```python
from build123d import *

# Parameters (mm, degrees)
SKETCH1_R                               = 87.47125
BOSS_EXTRUDE1_DEPTH                     = 25.4
BOSS_EXTRUDE2_DEPTH                     = 25.4
CUT_EXTRUDE1_REACH                      = 31.21
CUT_EXTRUDE1_START                      = -3.81
SKETCH8_R                               = 72.38365
CBORE_FOR_M6_HEX_HEAD_BOLT1_D           = 7
CBORE_FOR_M6_HEX_HEAD_BOLT1_CBORE_D     = 14.547
CBORE_FOR_M6_HEX_HEAD_BOLT1_CBORE_DEPTH = 4


with BuildPart() as part:
    # Sketch1 → Boss-Extrude1 (new body)
    with BuildSketch(Plane.XY):
        Circle(SKETCH1_R)
    extrude(amount=BOSS_EXTRUDE1_DEPTH)

    # Sketch3 → Boss-Extrude2 (add)
    with BuildSketch(Plane.XY):
        with BuildLine():
            ThreePointArc((-76.246005737, 105.719498865), (-102.262666579, 102.262666579), (-105.719498865, 76.246005737))
            ThreePointArc((-105.719498865, 76.246005737), (-92.490752346, 39.105377809), (-87.47125, 0))
            ThreePointArc((-87.47125, 0), (-92.490752346, -39.105377809), (-105.719498865, -76.246005737))
            ThreePointArc((-105.719498865, -76.246005737), (-102.262666579, -102.262666579), (-76.246005737, -105.719498865))
            ThreePointArc((-76.246005737, -105.719498865), (-39.105377809, -92.490752346), (0, -87.47125))
            ThreePointArc((0, -87.47125), (39.105377809, -92.490752346), (76.246005737, -105.719498865))
            ThreePointArc((76.246005737, -105.719498865), (102.262666579, -102.262666579), (105.719498865, -76.246005737))
            ThreePointArc((105.719498865, -76.246005737), (92.490752346, -39.105377809), (87.47125, 0))
            ThreePointArc((87.47125, 0), (92.490752346, 39.105377809), (105.719498865, 76.246005737))
            ThreePointArc((105.719498865, 76.246005737), (102.262666579, 102.262666579), (76.246005737, 105.719498865))
            ThreePointArc((76.246005737, 105.719498865), (39.105377809, 92.490752346), (0, 87.47125))
            ThreePointArc((0, 87.47125), (-39.105377809, 92.490752346), (-76.246005737, 105.719498865))
        make_face()
    extrude(amount=BOSS_EXTRUDE2_DEPTH)

    # Sketch8 → Cut-Extrude1 (cut, up to next)
    with BuildSketch(Plane.XY.offset(25.4).offset(CUT_EXTRUDE1_START), mode=Mode.PRIVATE) as cut_extrude1_sk1:
        Circle(SKETCH8_R)
    cut_extrude1_tool1 = extrude(cut_extrude1_sk1.sketch, amount=-CUT_EXTRUDE1_REACH, mode=Mode.PRIVATE) & part.part
    add(cut_extrude1_tool1.solids().sort_by_distance((0, 0, 21.59))[0], mode=Mode.SUBTRACT)

    # CBORE for M6 Hex Head Bolt1 (through all)
    with Locations(Plane.XY.offset(25.4)):
        with Locations((-86.996231173, 86.996231173), (86.996231173, 86.996231173), (86.996231173, -86.996231173), (-86.996231173, -86.996231173)):
            CounterBoreHole(CBORE_FOR_M6_HEX_HEAD_BOLT1_D / 2, CBORE_FOR_M6_HEX_HEAD_BOLT1_CBORE_D / 2, CBORE_FOR_M6_HEX_HEAD_BOLT1_CBORE_DEPTH)


solid = part.part
```
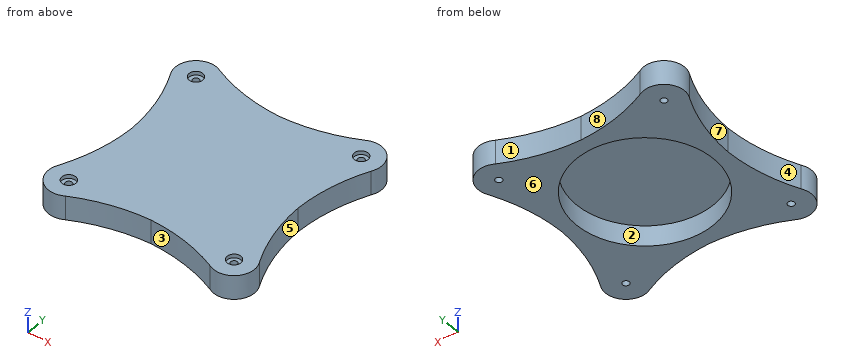
Design review of the part built by this model. Coordinates are the model's own, in mm. Face numbers are marked on the shaded views. A direction names the side the tool comes from. Coordinates: 2 decimals unless noted, no trailing zeros. Loops run counter-clockwise (first coordinate to the right, second up) from the corner with the lowest first, then second, coordinate; pieces in that order, holes last.
Q1. We need section B-B on x = 14.5. State the section outline as (y, z) points, and give its area (3 significant figures).
Reported:
outline: (-88.34, 0) - (-70.92, 0) - (-70.92, 21.59) - (70.92, 21.59) - (70.92, 0) - (88.34, 0) - (88.34, 25.4) - (-88.34, 25.4) - close
area: 1,430 mm2
Q2. We need section A-A on y = 5. State the section outline as (x, z) points, and give its area (3 significant figures).
Reported:
outline: (-87.64, 0) - (-72.21, 0) - (-72.21, 21.59) - (72.21, 21.59) - (72.21, 0) - (87.64, 0) - (87.64, 25.4) - (-87.64, 25.4) - close
area: 1,330 mm2
Q3. Tool access review of the marked faces 1, 2, 3, 4 and 5: name each direction out of +Z, -Z, +X, -X, +Y, -Y from which nothing blocks a thin tool from reaching the whole face with its end or side.
Reported:
face 1: +Z, -Z, +Y
face 2: -Z
face 3: +Z, -Z, -Y
face 4: +Z, -Z, -X
face 5: +Z, -Z, +X
Q4. To check wall thickness, follow line 1 (Z direction, x = -3, y = 1.5); line 2 (Y direction, x = 26.5, z = 14.5); line 3 (X direction, y = 58.5, z = 6). State the ranges of each line that lie inside material, in increasing order.
Reported:
line 1: z = 21.59 to 25.4
line 2: y = -89.94 to -67.36, 67.36 to 89.94
line 3: x = -98.28 to -42.63, 42.63 to 98.28
Q5. For pin 1 (1.5 mm diameter, centred on y = -11, z = 9.5, fed in from -X); pin 2 (5 mm diameter, centred on x = -26.5, z = 3, fed in from +Y); pin 3 (8 mm diameter, centred on x = 87, y = -87, fed in from +Z), all flat-tipped, find the tip position at first contact; note any pin that passes through.
Reported:
pin 1: stops at x = -88.09
pin 2: stops at y = 90.37
pin 3: stops at z = 21.4
Q6. The part is to be moulded in two halves that separate along X. For the marked faces 6, 7 and 8, say which applies: +X half, -X half, draft (parallel to the pull), parting line (faces both ways), or undercut.
Reported:
face 6: draft
face 7: -X half
face 8: undercut
Q7. We need section C-C on z = 4.5. State the section outline as (x, y) points.
Reported:
outline: (-105.72, -76.25) arc R21.59 ccw to (-76.25, -105.72) arc R184.15 cw to (0, -87.47) arc R184.15 cw to (76.25, -105.72) arc R21.59 ccw to (105.72, -76.25) arc R184.15 cw to (87.47, 0) arc R184.15 cw to (105.72, 76.25) arc R21.59 ccw to (76.25, 105.72) arc R184.15 cw to (0, 87.47) arc R184.15 cw to (-76.25, 105.72) arc R21.59 ccw to (-105.72, 76.25) arc R184.15 cw to (-87.47, 0) arc R184.15 cw to start; hole circle Ø7 at (-87, -87); hole circle Ø7 at (-87, 87); hole circle Ø144.77 at (0, 0); hole circle Ø7 at (87, -87); hole circle Ø7 at (87, 87)
